```python
from build123d import *

# Parameters (mm, degrees)
BOSS_EXTRUDE1_DEPTH = 12
CUT_EXTRUDE1_DEPTH  = 12


with BuildPart() as part:
    # Sketch1 → Boss-Extrude1 (new body)
    with BuildSketch(Plane(origin=(0, 0, 0), x_dir=(1, 0, 0), z_dir=(0, 1, 0))):
        with BuildLine():
            Line((-97, -75), (97, -75))
            ThreePointArc((97, -75), (99.121320344, -74.121320344), (100, -72))
            Line((100, -72), (100, 72))
            ThreePointArc((100, 72), (99.121320344, 74.121320344), (97, 75))
            Line((97, 75), (-97, 75))
            ThreePointArc((-97, 75), (-99.121320344, 74.121320344), (-100, 72))
            Line((-100, 72), (-100, -72))
            ThreePointArc((-100, -72), (-99.121320344, -74.121320344), (-97, -75))
        make_face()
    extrude(amount=BOSS_EXTRUDE1_DEPTH)

    # Sketch2 → Cut-Extrude1 (cut)
    with BuildSketch(Plane(origin=(0, 12, 0), x_dir=(1, 0, 0), z_dir=(0, 1, 0))):
        Polygon((-24.855906811, 48.549939904), (-11.856976443, 23.007043942), (-17.732961605, 7.632856116), (-30.731891973, 33.175752078), (-55.995225818, -32.924353512), (-69.695225818, -32.924353512), (-38.555906811, 48.549939904), align=None)
        Polygon((45.817241453, -8.158042149), (58.420963339, -32.924353512), (44.720963339, -32.924353512), (39.651548235, -22.962953695), (26.998770847, -53.344492874), (13.298770847, -53.344492874), (-3.795083958, -19.755071091), (2.080901204, -4.380883265), (19.464464064, -38.539581328), (32.117241453, -8.158042149), (11.082229848, 33.175752078), (-14.181103997, -32.924353512), (-27.881103997, -32.924353512), (3.25821501, 48.549939904), (16.95821501, 48.549939904), (38.28293467, 6.646869398), (46.899276911, 27.336219357), (60.599276911, 27.336219357), align=None)
    extrude(amount=-CUT_EXTRUDE1_DEPTH, mode=Mode.SUBTRACT)


solid = part.part
```
Work out the finished part from the listing and answer in its coordinate system (mm). Give positions to 0.01 mm unless a question says otherwise; leave off trailing zeros. Write each loop counter-clockwise with the first axis right and the second up, starting at its lowest first coordinate (ties: lowest second). Pieces come first, ordered by that corner, then holes.
(1) The mould has two halves that part along Z. Classify faces 1 (the flat face through (-100, 6, -1)), 2 (the flat face through (21.747, 6.084, -12.22)), 3 (the flat face through (1, 6, -75)): pulls with the +Z half, pulls with the -Z half, needs draft (parallel to the pull), parting line crosses it, or undercut.
Final values:
face 1: needs draft
face 2: undercut
face 3: pulls with the -Z half
(2) The part is cut by section A-A on y = 8.5. Count the separate pieces of the cut face and the enclosed holes in it, plus the area to 3 significant figures.
Final values:
separate pieces: 1
enclosed holes: 2
area: 25,000 mm2
(3) The part is cut by section D-D on x = 6. Write down the section's boundary in (y, z), plus the area to 3 significant figures.
Final values:
outline: (0, -75) - (12, -75) - (12, -48.55) - (0, -48.55) - close; (0, -19.88) - (12, -19.88) - (12, 12.08) - (0, 12.08) - close; (0, 39) - (12, 39) - (12, 75) - (0, 75) - close
area: 1,130 mm2
(4) Straight lines are drawn through the part: line 1 (X direction, y = 9.5, z = -39); line 2 (X direction, y = 9, z = 8); line 3 (X direction, y = 9.5, z = -48). For each, find the intervals that lie inside material, in ascending order.
Final values:
line 1: x = -100 to -42.21, -20 to -0.39, 21.82 to 100
line 2: x = -100 to -60.17, -46.47 to -18.36, -4.66 to 0.7, 3.92 to 32.04, 45.88 to 100
line 3: x = -100 to -38.77, -24.58 to 3.05, 17.24 to 100
(5) The part is cut by section B-B on z = 17. Write down the section's boundary in (x, y), plus the area to 3 significant figures.
Final values:
outline: (-100, 0) - (-63.61, 0) - (-63.61, 12) - (-100, 12) - close; (-49.91, 0) - (-21.79, 0) - (-21.79, 12) - (-49.91, 12) - close; (-8.09, 0) - (-2.74, 0) - (-2.74, 12) - (-8.09, 12) - close; (8.5, 0) - (28.43, 0) - (28.43, 12) - (8.5, 12) - close; (50.32, 0) - (100, 0) - (100, 12) - (50.32, 12) - close
area: 1,670 mm2
(6) The part is cut by section C-C on z = -45.5. Write down the section's boundary in (x, y).
Final values:
outline: (-100, 0) - (-39.72, 0) - (-39.72, 12) - (-100, 12) - close; (-23.3, 0) - (2.09, 0) - (2.09, 12) - (-23.3, 12) - close; (18.51, 0) - (100, 0) - (100, 12) - (18.51, 12) - close
